```python
from build123d import *

# Parameters (mm, degrees)
SHELL_DEPTH                       = 43
SK_TABS_W                         = 9.6
SK_TABS_H                         = 12
MOUNTING_TABS_DEPTH               = 43
SK_CAVITY_W                       = 128
SK_CAVITY_H                       = 51
CAVITY_DEPTH                      = 159.137408604
SK_LIP_W                          = 128
SK_LIP_H                          = 51
SK_LIP_W_2                        = 124
SK_LIP_H_2                        = 47
BOARD_LIP_DEPTH                   = 2
SK_RAILS_W                        = 2
SK_RAILS_H                        = 48
BOARD_RAILS_DEPTH                 = 1.5
SK_SLOTA_W                        = 15
SK_SLOTA_H                        = 10
CABLE_SLOT_15X10_DEPTH            = 3
SK_SLOTB_W                        = 18
SK_SLOTB_H                        = 10
CABLE_SLOT_18X10_DEPTH            = 3
TAB_M3_CLEARANCE_HOLES_DEPTH      = 159.872275744
TAB_M3_CLEARANCE_HOLES_DEPTH_BACK = 159.872275744
SK_TABHOLES_R                     = 1.7
SK_FLOORHOLES_R                   = 1.7
FLOOR_M3_CLEARANCE_HOLES_DEPTH    = 2.8
SK_CBORE_R                        = 3.4
FLOOR_COUNTERBORES_DEPTH          = 1


with BuildPart() as part:
    # Sk_Shell → Shell (new body)
    with BuildSketch(Plane(origin=(0, 0, 0), x_dir=(1, 0, 0), z_dir=(0, 1, 0))):
        with BuildLine():
            Line((4, 0), (128.8, 0))
            ThreePointArc((128.8, 0), (131.628427125, 1.171572875), (132.8, 4))
            Line((132.8, 4), (132.8, 51.8))
            ThreePointArc((132.8, 51.8), (131.628427125, 54.628427125), (128.8, 55.8))
            Line((128.8, 55.8), (4, 55.8))
            ThreePointArc((4, 55.8), (1.171572875, 54.628427125), (0, 51.8))
            Line((0, 51.8), (0, 4))
            ThreePointArc((0, 4), (1.171572875, 1.171572875), (4, 0))
        make_face()
    extrude(amount=SHELL_DEPTH)

    # Sk_Tabs → Mounting Tabs (add)
    with BuildSketch(Plane(origin=(0, 0, 0), x_dir=(1, 0, 0), z_dir=(0, 1, 0))):
        with Locations((-4.8, 12)):
            Rectangle(SK_TABS_W, SK_TABS_H)
        with Locations((137.6, 12)):
            Rectangle(SK_TABS_W, SK_TABS_H)
        with Locations((-4.8, 43.8)):
            Rectangle(SK_TABS_W, SK_TABS_H)
        with Locations((137.6, 43.8)):
            Rectangle(SK_TABS_W, SK_TABS_H)
    extrude(amount=MOUNTING_TABS_DEPTH)

    # Sk_Cavity → Cavity (cut, through all)
    with BuildSketch(Plane(origin=(0, 2.8, 0), x_dir=(1, 0, 0), z_dir=(0, 1, 0))):
        with Locations((66.4, 27.9)):
            Rectangle(SK_CAVITY_W, SK_CAVITY_H)
    extrude(amount=CAVITY_DEPTH, mode=Mode.SUBTRACT)

    # Sk_Lip → Board Lip (add)
    with BuildSketch(Plane(origin=(0, 4, 0), x_dir=(1, 0, 0), z_dir=(0, 1, 0))):
        with Locations((66.4, 27.9)):
            Rectangle(SK_LIP_W, SK_LIP_H)
        with Locations((66.4, 27.9)):
            Rectangle(SK_LIP_W_2, SK_LIP_H_2, mode=Mode.SUBTRACT)
    extrude(amount=BOARD_LIP_DEPTH)

    # Sk_Rails → Board Rails (add)
    with BuildSketch(Plane(origin=(0, 6, 0), x_dir=(1, 0, 0), z_dir=(0, 1, 0))):
        with Locations((4.9, 27.9)):
            Rectangle(SK_RAILS_W, SK_RAILS_H)
        with Locations((127.9, 27.9)):
            Rectangle(SK_RAILS_W, SK_RAILS_H)
    extrude(amount=BOARD_RAILS_DEPTH)

    # Sk_SlotA → Cable Slot 15x10 (cut)
    with BuildSketch(Plane(origin=(0, 0, 0), x_dir=(0, 0, -1), z_dir=(1, 0, 0))):
        with Locations((27.9, 11)):
            Rectangle(SK_SLOTA_W, SK_SLOTA_H)
    extrude(amount=CABLE_SLOT_15X10_DEPTH, mode=Mode.SUBTRACT)

    # Sk_SlotB → Cable Slot 18x10 (cut)
    with BuildSketch(Plane(origin=(132.8, 0, 0), x_dir=(0, 0, -1), z_dir=(1, 0, 0))):
        with Locations((27.9, 11)):
            Rectangle(SK_SLOTB_W, SK_SLOTB_H)
    extrude(amount=-CABLE_SLOT_18X10_DEPTH, mode=Mode.SUBTRACT)

    # Sk_TabHoles → Tab M3 Clearance Holes (cut, two sides: drawn at the far end of the back side and taken through both)
    with BuildSketch(Plane(origin=(0, 0, 0), x_dir=(1, 0, 0), z_dir=(0, 1, 0)).offset(-TAB_M3_CLEARANCE_HOLES_DEPTH_BACK)):
        with Locations(Location((-3.6, 12, 0), (0, 0, 270))):
            Circle(SK_TABHOLES_R)
        with Locations(Location((-3.6, 43.8, 0), (0, 0, 270))):
            Circle(SK_TABHOLES_R)
        with Locations(Location((136.4, 12, 0), (0, 0, 270))):
            Circle(SK_TABHOLES_R)
        with Locations(Location((136.4, 43.8, 0), (0, 0, 270))):
            Circle(SK_TABHOLES_R)
    extrude(amount=TAB_M3_CLEARANCE_HOLES_DEPTH + TAB_M3_CLEARANCE_HOLES_DEPTH_BACK, mode=Mode.SUBTRACT)

    # Sk_FloorHoles → Floor M3 Clearance Holes (cut)
    with BuildSketch(Plane(origin=(0, 0, 0), x_dir=(1, 0, 0), z_dir=(0, 1, 0))):
        with Locations(Location((5.9, 5.9, 0), (0, 0, 270))):
            Circle(SK_FLOORHOLES_R)
        with Locations(Location((126.9, 5.9, 0), (0, 0, 270))):
            Circle(SK_FLOORHOLES_R)
        with Locations(Location((5.9, 49.9, 0), (0, 0, 270))):
            Circle(SK_FLOORHOLES_R)
        with Locations(Location((126.9, 49.9, 0), (0, 0, 270))):
            Circle(SK_FLOORHOLES_R)
    extrude(amount=FLOOR_M3_CLEARANCE_HOLES_DEPTH, mode=Mode.SUBTRACT)

    # Sk_CBore → Floor Counterbores (cut)
    with BuildSketch(Plane(origin=(0, 2.8, 0), x_dir=(1, 0, 0), z_dir=(0, 1, 0))):
        with Locations(Location((5.9, 5.9, 0), (0, 0, 270))):
            Circle(SK_CBORE_R)
        with Locations(Location((126.9, 5.9, 0), (0, 0, 270))):
            Circle(SK_CBORE_R)
        with Locations(Location((5.9, 49.9, 0), (0, 0, 270))):
            Circle(SK_CBORE_R)
        with Locations(Location((126.9, 49.9, 0), (0, 0, 270))):
            Circle(SK_CBORE_R)
    extrude(amount=-FLOOR_COUNTERBORES_DEPTH, mode=Mode.SUBTRACT)


solid = part.part
```
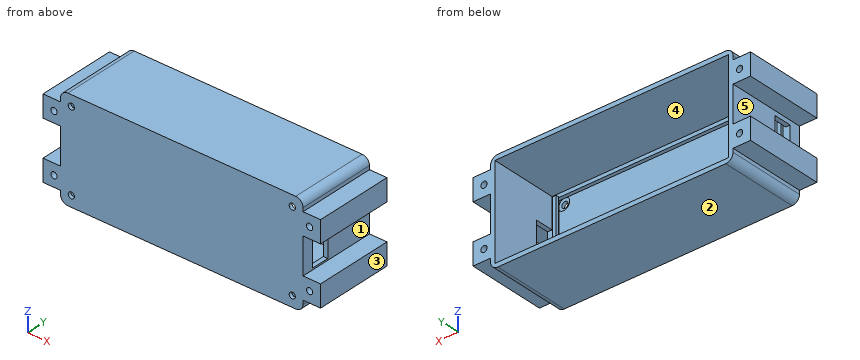
For this review, take the finished solid that the model builds, in its own axes (mm). Face numbers are marked on the shaded views. A direction names the side the tool comes from. Coordinates: 2 decimals unless noted, no trailing zeros. Order: outer loops, then holes, each group sorted by start corner. A loop starts at its lowest first (then second) coordinate and runs counter-clockwise, first axis right, second up. Notation, with made-up numbers: (78, 60.5) -> (93, 60.5) arc R14 ccw to (93, 74.5) -> close; hole circle Ø6 at (41.25, 89). An arc over 180 degrees is marked (long way). Use CSV: the item, a comma, the result in double quotes. Start each with the question number.
Item 1: We need section D-D, the plane x = 112. Give the boundary of the cut face in (y, z).
Item 2: Insertion check: pin 1 (4 mm diameter, centred on y = 34.5, z = -22, fed in from -X); pin 2 (4 mm diameter, centred on x = 78, z = -25, fed in from +Y); pin 3 (2.5 mm diameter, centred on x = 126.9, z = -49.9, fed in from +Y); pin 4 (2 mm diameter, centred on x = -3.6, z = -12, fed in from +Y). Each pin has a flat end and moves straight along its axis. Give the tip position at first contact, or say it passes through.
Item 3: For the marked faces 1, 2, 3, 4 and 5, list the 3-axis set-ups (+Z, -Z, +X, -X, +Y, -Y) from which the entire face can be reached by the end or side of a thin tool; tool diameter is ignored.
Item 4: Wall thickness on probe 1 along Z at (x, y) = (126.9, 0.75); probe 2 along Z at (x, y) = (136.4, 19); probe 3 along X at (y, z) = (1.4, -5.9): over which ranges is each line inside the solid? List them lowest first.
Item 5: We need section A-A, the plane x = 136.4. Give the boundary of the cut face in (y, z), then the cut area to 3 significant figures.
Item 6: We need section B-B, the plane z = -43.8. Give the number of separate pieces and of enclosed holes in the cut face, then the cut area to 3 significant figures.
Derived:
1,outline,"(0, -55.8) -> (43, -55.8) -> (43, -53.4) -> (6, -53.4) -> (6, -51.4) -> (4, -51.4) -> (4, -53.4) -> (2.8, -53.4) -> (2.8, -2.4) -> (4, -2.4) -> (4, -4.4) -> (6, -4.4) -> (6, -2.4) -> (43, -2.4) -> (43, 0) -> (0, 0) -> close"
2,pin 1,"stops at x = 0"
2,pin 2,"stops at y = 2.8"
2,pin 3,"stops at y = 7.5"
2,pin 4,"passes through"
3,face 1,"+X, +Y, -Y"
3,face 2,"-Z, +X, -X, +Y, -Y"
3,face 3,"+Z, -Z, +X, +Y, -Y"
3,face 4,"+Y"
3,face 5,"-X, +Y, -Y"
4,probe 1,"z = -55.8 to -51.6, -48.2 to -7.6, -4.2 to 0"
4,probe 2,"z = -49.8 to -45.5, -42.1 to -37.8, -18 to -13.7, -10.3 to -6"
4,probe 3,"x = 0 to 4.2, 7.6 to 125.2, 128.6 to 132.8"
5,outline,"(0, -49.8) -> (43, -49.8) -> (43, -45.5) -> (0, -45.5) -> close; (0, -42.1) -> (43, -42.1) -> (43, -37.8) -> (0, -37.8) -> close; (0, -18) -> (43, -18) -> (43, -13.7) -> (0, -13.7) -> close; (0, -10.3) -> (43, -10.3) -> (43, -6) -> (0, -6) -> close"
5,area,"740 mm^2"
6,separate pieces,"3"
6,enclosed holes,"0"
6,area,"1,110 mm^2"
